Geometry: final body of the model. Coordinates: model frame, mm. Give positions to 0.01 mm unless a question says otherwise; leave off trailing zeros. Order: outer loops, then holes, each group sorted by start corner. A loop starts at its lowest first (then second) coordinate and runs counter-clockwise, first axis right, second up. Notation, with made-up numbers: (55, 9.5) - (89, 9.5) arc R34 ccw to (89, 43.5) - close; hole circle Ø6 at (51, -24.75). An arc over 180 degrees is marked (long way). One line per item, written item: value.
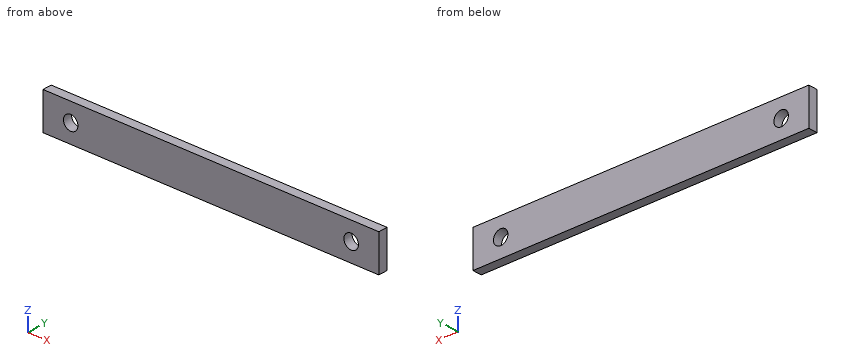
Autodesk Inventor part; units mm, degrees
ref_plane "YZ Plane" through (0, 0, 0) normal (1, 0, 0) x (0, 1, 0)
ref_plane "XZ Plane" through (0, 0, 0) normal (0, 1, 0) x (-1, 0, 0)
ref_plane "XY Plane" through (0, 0, 0) normal (0, 0, 1) x (1, 0, 0)
sketch "Sketch2" plane through (0, 0, 0) normal (0, 1, 0) x (-1, 0, 0)
  line L0 (0, 0) -> (-115.5161, 0)
  line L1 (-115.5161, 0) -> (-115.5161, -12.7)
  line L2 (-115.5161, -12.7) -> (0, -12.7)
  line L3 (0, -12.7) -> (0, 0)
  line L4 (0, -6.35) -> (-115.5161, -6.35)
  point P0 (-9.525, -6.35)
  point P1 (-105.9911, -6.35)
  dimension "d12" = 12.7
  dimension "d13" = 9.525
  dimension "d14" = 9.525
  dimension "d15" = 96.4661
extrude "Extrusion2" add sketch "Sketch2" along normal blind 3.175
hole "Hole2" at (9.525, 0, -6.35) at (105.9911, 0, -6.35) direction (0, 1, 0) diameter 4.9784 end through all
equation "\"height\" = 203.2"
equation "\"thickness\" = 12.7"
equation "\"shaftDiam\" = 6.35"
equation "\"shaftSpace\" = 1.5875"
equation "\"stageSpace\" = 2.54"
equation "\"stageAngle\" = 15deg"
equation "\"bearingDiam\" = 9.5504"
equation "\"FlangeDiam\" = 12.7"
equation "\"FlangeDepth\" = 1.5875"
equation "\"smallFilet\" = 0.39687"
equation "\"ringDiam\" = 96.46608"
equation "\"stockHeight\" = 50.8"
equation "\"stockWidth\" = 76.2"
equation "\"stockRad\" = 9.525"
equation "\"stockGuage\" = 3.175"
equation "\"groundActu\" = 304.8"
equation "\"baseWidth\" = 1066.8"
equation "\"baseDepth\" = 254"
equation "\"capThickness\" = 3.175"
equation "\"sup1Len\" = 660.4"
equation "\"sup1Ang\" = 22.619865deg"
equation "\"sup2Len\" = 2079.37366"
equation "\"sup2Ang\" = 8.959949deg"
equation "\"supVertLen\" = 955.13561"
equation "\"supSideLen\" = 1531.12879"
equation "\"supSideAng\" = 19.376933deg"
properties part number "lock ring 1 supp" material "Aluminum 6061"
1) First-contact query: pin 1 (4 mm diameter, centred on x = 86.5, z = -2.5, fed in from -Y). Flat tip, straight axial feed; report the tip coordinate or a pass-through.
Answers below:
pin 1: y = 0
2) Material intervals for line 1 along X through (y, z) = (1.95, -6.35); line 2 along X through (y, z) = (1.5, -7.5), sorted ascending.
Answers below:
line 1: 0 to 7.04, 12.01 to 103.5, 108.48 to 115.52
line 2: 0 to 7.32, 11.73 to 103.78, 108.2 to 115.52
3) Section A-A, the plane z = -6.35. Return loops of the section in (x, y) (3 decimals), then the cut area to 3 significant figures.
Answers below:
outline: (0, 0) - (7.036, 0) - (7.036, 3.175) - (0, 3.175) - close; (12.014, 0) - (103.502, 0) - (103.502, 3.175) - (12.014, 3.175) - close; (108.48, 0) - (115.516, 0) - (115.516, 3.175) - (108.48, 3.175) - close
area: 335 mm^2
4) Section B-B, the plane y = 2.05. Return loops of the section in (x, z) (3 decimals), then the cut area to 3 significant figures.
Answers below:
outline: (0, -12.7) - (115.516, -12.7) - (115.516, 0) - (0, 0) - close; hole circle Ø4.978 at (9.525, -6.35); hole circle Ø4.978 at (105.991, -6.35)
area: 1,430 mm^2
